Model file for the job. Use its own axes, mm. Round coordinates to 2 decimals unless told otherwise and drop trailing zeros. Loops run counter-clockwise (first coordinate to the right, second up) from the corner with the lowest first, then second, coordinate; pieces in that order, holes last. Notation, with made-up numbers: M -0.5,59.25 L 44.5,59.25 A26 ccw 44.5,91.25 Z; hole C -25.5,-17.5 d8. An arc over 180 degrees is marked long. Use a Markdown table: item, result. Add a question column.
Q1. Pin check, flat tips, straight feed: pin 1 (1.5 mm diameter, centred on x = 113, y = 76, fed in from +Z); pin 2 (5 mm diameter, centred on x = 90.5, z = 9, fed in from -Y); pin 3 (1 mm diameter, centred on x = 154, z = 6.5, fed in from -Y); pin 4 (2 mm diameter, centred on x = 150, y = 73, fed in from -Z). Stop position of each tip, or through.
Q2. Cut at A-A (y = 69.5). Give the cut face in (x, z), plus the area to 3 significant figures.
Q3. Probe line 1 (X direction, y = 84.5, z = 5.25); line 2 (X direction, y = 88, z = 12.25); line 3 (Z direction, x = 109, y = 39). List the from-to ranges inside material, lowest first. Write a range as from..to.
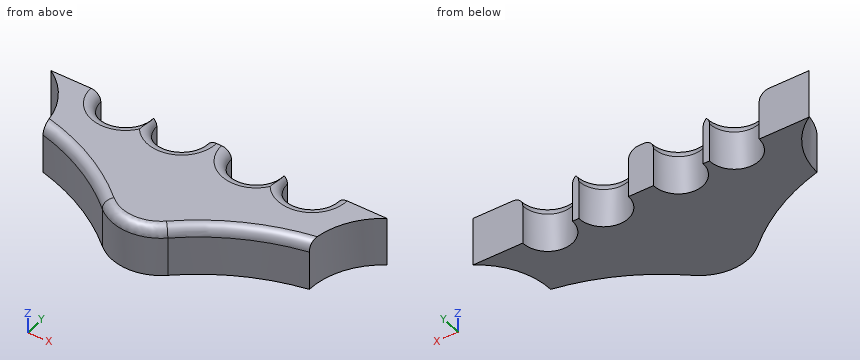
from build123d import *

# Parameters (mm, degrees)
F1_DEPTH    = 25.4
F2_R        = 25.4
F3_T2_ANGLE = 294.7758439205
F3_T4_ANGLE = 294.7758439205
F3_T6_ANGLE = 294.7758439205
F3_T8_ANGLE = 294.7758439205
F4_R        = 5.08


# Not quite as in the source:
# - a fillet or chamfer that OpenCascade refuses, or shapes differently, is made with other operations: its cross-section is extruded or revolved along the edge and cut away or added


with BuildPart() as f1:
    # F0 (on Top) → F1 (new body)
    with BuildSketch(Plane.XY):
        with BuildLine():
            Line((37.1146484218, 92.3934370832), (11.7146484218, 92.3934370832))
            ThreePointArc((11.7146484218, 92.3934370832), (24.640162726, 78.7783250935), (29.4946484218, 60.6434370832))
            ThreePointArc((29.4946484218, 60.6434370832), (65.749840409, 44.0578596931), (94.2646484218, 16.1934370832))
            ThreePointArc((94.2646484218, 16.1934370832), (125.6004493922, 45.1771555306), (165.3846484218, 60.6434370832))
            ThreePointArc((165.3846484218, 60.6434370832), (170.2391341176, 78.7783250935), (183.1646484218, 92.3934370832))
            Line((183.1646484218, 92.3934370832), (157.7646484218, 92.3934370832))
            ThreePointArc((157.7646484218, 92.3934370832), (145.0646484218, 79.6934370832), (132.3646484218, 92.3934370832))
            Line((132.3646484218, 92.3934370832), (129.1896484218, 92.3934370832))
            ThreePointArc((129.1896484218, 92.3934370832), (116.4896484218, 79.6934370832), (103.7896484218, 92.3934370832))
            Line((103.7896484218, 92.3934370832), (91.0896484218, 92.3934370832))
            ThreePointArc((91.0896484218, 92.3934370832), (78.3896484218, 79.6934370832), (65.6896484218, 92.3934370832))
            Line((65.6896484218, 92.3934370832), (62.5146484218, 92.3934370832))
            ThreePointArc((62.5146484218, 92.3934370832), (49.8146484218, 79.6934370832), (37.1146484218, 92.3934370832))
        make_face()
    extrude(amount=F1_DEPTH)

    # F2
    f2_edges = [f1.edges().sort_by_distance(p)[0] for p in [
        (94.264648, 16.193437, 12.7),
    ]]
    fillet(f2_edges, radius=F2_R)

    # F3: fillet of radius 5.08 on 4 edges, made by hand

    # F3_s1 → F3_t2 (revolve, cut)
    with BuildSketch(Plane(origin=(-6.5992867665, 4.2223803326, 0), x_dir=(0, 0, 1), z_dir=(-0.8423388046, 0.5389483633, 0))):
        with BuildLine():
            ThreePointArc((25.4, 122.4541005786), (23.9121024484, 118.8619981302), (20.32, 117.3741005786))
            Line((20.32, 117.3741005786), (25.4, 117.3741005786))
            Line((25.4, 117.3741005786), (25.4, 122.4541005786))
        make_face()
    revolve(axis=Axis((49.8146484218, 92.3934370832, 25.4), (0, 0, -1)), revolution_arc=F3_T2_ANGLE, mode=Mode.SUBTRACT)

    # F3_s3 → F3_t4 (revolve, cut)
    with BuildSketch(Plane(origin=(40.7089368011, -26.0465441486, 0), x_dir=(0, 0, 1), z_dir=(-0.8423388046, 0.5389483633, 0))):
        with BuildLine():
            ThreePointArc((25.4, 158.3884827026), (23.9121024484, 154.7963802542), (20.32, 153.3084827026))
            Line((20.32, 153.3084827026), (25.4, 153.3084827026))
            Line((25.4, 153.3084827026), (25.4, 158.3884827026))
        make_face()
    revolve(axis=Axis((116.4896484218, 92.3934370832, 25.4), (0, 0, -1)), revolution_arc=F3_T4_ANGLE, mode=Mode.SUBTRACT)

    # F3_s5 → F3_t6 (revolve, cut)
    with BuildSketch(Plane(origin=(60.9838897586, -39.0189403548, 0), x_dir=(0, 0, 1), z_dir=(-0.8423388046, 0.5389483633, 0))):
        with BuildLine():
            ThreePointArc((25.4, 173.7889321843), (23.9121024484, 170.1968297359), (20.32, 168.7089321843))
            Line((20.32, 168.7089321843), (25.4, 168.7089321843))
            Line((25.4, 168.7089321843), (25.4, 173.7889321843))
        make_face()
    revolve(axis=Axis((145.0646484218, 92.3934370832, 25.4), (0, 0, -1)), revolution_arc=F3_T6_ANGLE, mode=Mode.SUBTRACT)

    # F3_s7 → F3_t8 (revolve, cut)
    with BuildSketch(Plane(origin=(13.6756661911, -8.7500158736, 0), x_dir=(0, 0, 1), z_dir=(-0.8423388046, 0.5389483633, 0))):
        with BuildLine():
            ThreePointArc((25.4, 137.8545500603), (23.9121024484, 134.2624476119), (20.32, 132.7745500603))
            Line((20.32, 132.7745500603), (25.4, 132.7745500603))
            Line((25.4, 132.7745500603), (25.4, 137.8545500603))
        make_face()
    revolve(axis=Axis((78.3896484218, 92.3934370832, 25.4), (0, 0, -1)), revolution_arc=F3_T8_ANGLE, mode=Mode.SUBTRACT)

    # F4
    f4_edges = [f1.edges().sort_by_distance(p)[0] for p in [
        (94.329479, 28.280902, 25.4),
    ]]
    fillet(f4_edges, radius=F4_R)


with BuildPart() as f5_1:
    # F5: copy of F1
    add(f1.part)


with BuildPart() as f6_1:
    # F6: copy of F5_1
    add(f5_1.part.moved(Location((0, 0, 50.8))))


solid = f1.part
Checked values:
| question | item | result |
|---|---|---|
| 1 | pin 1 | stops at z = 25.39 |
| 1 | pin 2 | stops at y = 28.33 |
| 1 | pin 3 | stops at y = 57.78 |
| 1 | pin 4 | stops at z = 0 |
| 2 | outline | M 28.34,0 L 166.54,0 L 166.54,25.4 L 28.34,25.4 Z |
| 2 | area | 3,510 mm^2 |
| 3 | line 1 | x = 20.71..39.87, 59.76..68.44, 88.34..106.54, 126.44..135.12, 155.01..174.17 |
| 3 | line 2 | x = 17.41..37.9, 61.73..66.47, 90.31..104.57, 128.41..133.15, 156.98..177.47 |
| 3 | line 3 | z = 0..25.39 |
